Input: part model. Units: mm. Frame: model coordinates. A direction names the side the tool comes from. Give positions to 0.01 mm unless a question says otherwise; leave off trailing zeros. Write each loop counter-clockwise with the first axis right and the second up, starting at its lowest first coordinate (ties: lowest second). Pieces come first, ordered by that corner, then holes.
Autodesk Inventor part; units mm, degrees
ref_plane "Work Plane1" through (0, 0, -18.5) normal (0, 0, -1) x (-1, 0, 0)
ref_plane "YZ Plane" through (0, 0, 0) normal (1, 0, 0) x (0, 1, 0)
ref_plane "XZ Plane" through (0, 0, 0) normal (0, 1, 0) x (-1, 0, 0)
sketch "Sketch1" plane through (0, 0, 0) normal (0, 0, 1) x (1, 0, 0)
  circle A0 centre (0, 0) radius 4.225
  dimension "d0" = 8.45
extrude "Extrusion1" add sketch "Sketch1" against normal blind 3
sketch "Sketch2" plane through (0, 0, -3) normal (0, 0, -1) x (-1, 0, 0)
  circle A0 centre (0, 0) radius 2.475
  dimension "d3" = 4.95
extrude "Extrusion2" add sketch "Sketch2" along normal blind 40
thread "Thread1"
sketch "Sketch3" plane through (0, 0, 0) normal (0, 0, 1) x (1, 0, 0)
  line L0 (-1.2124, -2.1) -> (-2.4249, 0)
  line L1 (-2.4249, 0) -> (-1.2124, 2.1)
  line L2 (-1.2124, 2.1) -> (1.2124, 2.1)
  line L3 (1.2124, 2.1) -> (2.4249, 0)
  line L4 (2.4249, 0) -> (1.2124, -2.1)
  line L5 (1.2124, -2.1) -> (-1.2124, -2.1)
  line L6 (-4.5, -0.75) -> (4.5, -0.75)
  line L7 (4.5, -0.75) -> (4.5, 0.75)
  line L8 (4.5, 0.75) -> (-4.5, 0.75)
  line L9 (-4.5, 0.75) -> (-4.5, -0.75)
  line L10 (-4.5, -0.75) -> (4.5, 0.75) construction
  line L11 (4.5, -0.75) -> (-4.5, 0.75) construction
  point P0 (0, 0)
  point P1 (0, 0)
  dimension "d8" = 2.1
  dimension "d13" = 4.2
  dimension "d18" = 9
  dimension "d19" = 1.5
extrude "Extrusion3" cut sketch "Sketch3" against normal blind 2 contours L0 L6 L4 L5 | L0 L1 L8 L3 L4 L6 | L1 L2 L3 L8
fillet "Fillet1" radius 0.5 2 edges at (-4.225, 0, 0) (-4.225, 0, -3)
ref_plane "Work Plane1" through (0, 0, -18.5) normal (0, 0, -1) x (-1, 0, 0)
sketch "Sketch4" plane through (0, 0, -43) normal (0, 0, -1) x (-1, 0, 0)
  circle A0 centre (0, 0) radius 2.475
extrude "Extrusion4" cut sketch "Sketch4" against normal blind 19
properties part number "ScrewM5x40_Machined" material "Aluminum 6061-AHC"
Item 1: Section B-B (z = -7.75). Return loops of the section in (x, y) (3 decimals), and give its area (3 significant figures).
Item 2: Set-up query: faces 1 (the flat face through (0, 0, -24)), 2 (the cylindrical face through (-2.36, -0.74, -13.35)), 3 (the flat face through (-1.827, 1.035, -0.986)). Return all of +Z, -Z, +X, -X, +Y, -Y with unobstructed straight access to the full face (end or side cutting, diameter ignored); none if empty.
Item 3: Mould query, pull axis Y, two halves, no side actions, for faces 4 (the cylindrical face through (4.03, 1.27, -1.49)), 5 (the flat face through (2, -2, 0)), 6 (the flat face through (-1.81, -1.065, -0.986)). Classes: +Y half, -Y half, draft (parallel to the pull), parting line (faces both ways), or undercut.
Item 4: Section A-A (x = 0). Return loops of the section in (y, z) (3 decimals).
Item 5: Pin query (flat end, axial travel): pin 1 (1.5 mm diameter, centred on x = -1, z = -7.5, fed in from -Y); pin 2 (3 mm diameter, centred on y = 1.5, z = -13, fed in from -X) (3 decimals); pin 3 (3 mm diameter, centred on x = 0, z = -15, fed in from +Y) (3 decimals). Return the tip coordinate at first contact, or that it passes through.
Item 6: Ray query, line 1 (Z direction, x = -2.5, y = 0.75); line 2 (Z direction, x = -1.75, y = -0.5); line 3 (Y direction, x = 1, z = -0.75). Return the intervals inside material, ascending.
Solved:
1. outline: circle Ø4.95 at (0, 0)
1. area: 19.2 mm2
2. face 1: -Z, +X, -X, +Y, -Y
2. face 2: -Z
2. face 3: +Z
3. face 4: parting line
3. face 5: draft
3. face 6: undercut
4. outline: (-4.225, -2.5) arc R0.5 ccw to (-3.725, -3) - (-2.475, -3) - (-2.475, -24) - (2.475, -24) - (2.475, -3) - (3.725, -3) arc R0.5 ccw to (4.225, -2.5) - (4.225, -0.5) arc R0.5 ccw to (3.725, 0) - (2.1, 0) - (2.1, -2) - (-2.1, -2) - (-2.1, 0) - (-3.725, 0) arc R0.5 ccw to (-4.225, -0.5) - close
5. pin 1: stops at y = -2.46
5. pin 2: stops at x = -2.475
5. pin 3: stops at y = 2.475
6. line 1: z = -3 to 0
6. line 2: z = -24 to -2
6. line 3: y = -4.1 to -2.1, 2.1 to 4.1
